Can you work these out from the model? Positions are in its coordinate system, mm. Face numbers are marked on the shaded views. A direction names the side the tool comes from. Give positions to 0.01 mm unless a question says otherwise; leave off trailing zeros. Loops run counter-clockwise (first coordinate to the right, second up) from the corner with the lowest first, then second, coordinate; pieces in that order, holes last. Notation, with made-up numbers: (-30.5, 9.25) -> (-15.5, 9.25) arc R29 cw to (-15.5, 45.25) -> close; hole circle Ø3 at (68, -5.75). An arc over 180 degrees is marked (long way). Use CSV: the item, a comma, the result in double quotes.
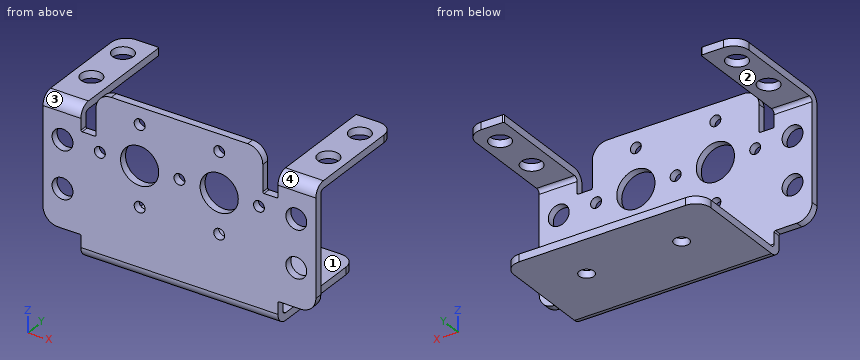
from build123d import *

# Parameters (mm, degrees)
BASE_FLANGE1_DEPTH             = 1.5494
EDGE_FLANGE1_STRIP_W           = 7.8232
EDGE_FLANGE1_STRIP_H           = 1.5494
EDGE_FLANGE1_STRIP_CUT_DEPTH   = 41.275
EDGE_FLANGE1_DEPTH             = 41.275
EDGE_FLANGE2_STRIP_W           = 7.8232
EDGE_FLANGE2_STRIP_H           = 1.5494
EDGE_FLANGE2_STRIP_CUT_DEPTH   = 7.9375
EDGE_FLANGE2_STRIP_2_W         = 7.8232
EDGE_FLANGE2_STRIP_2_H         = 1.5494
EDGE_FLANGE2_STRIP_CUT_2_DEPTH = 7.9375
EDGE_FLANGE2_DEPTH             = 7.9375
EDGE_FLANGE2_BEND_DEPTH        = 7.9375
SKETCH13_R                     = 1.143
SKETCH13_R_2                   = 4.0005
SKETCH13_R_3                   = 2.1844
EXTRUDE2_DEPTH                 = 1.5494
SKETCH14_R                     = 2.1844
EXTRUDE3_DEPTH                 = 1.5494
SKETCH15_R                     = 1.5621
EXTRUDE4_DEPTH                 = 1.5494
FILLET1_R                      = 3.175
FILLET2_R                      = 0.254


# Sheet-metal steps are written as plain solids
with BuildPart() as part:
    # Sketch1 → Base-Flange1 (new body)
    with BuildSketch(Plane(origin=(0, 0, 0), x_dir=(1, 0, 0), z_dir=(0, 1, 0))):
        Polygon((-17.4625, -11.8745), (17.4625, -11.8745), (17.4625, -2.9337), (20.6375, -2.9337), (20.6375, -6.3754), (28.575, -6.3754), (28.575, 17.8816), (20.6375, 17.8816), (20.6375, 21.3106), (-20.6375, 21.3106), (-20.6375, 17.8816), (-28.575, 17.8816), (-28.575, -6.3754), (-20.6375, -6.3754), (-20.6375, -2.9337), (-17.4625, -2.9337), align=None)
    extrude(amount=BASE_FLANGE1_DEPTH)

    # Edge-Flange1 strip (across the edge) → Edge-Flange1 strip cut (cut)
    with BuildSketch(Plane(origin=(20.6375, 1.5494, -21.3106), x_dir=(0, 0, 1), z_dir=(-1, 0, 0))):
        with Locations((-3.0988, -0.7747)):
            Rectangle(EDGE_FLANGE1_STRIP_W, EDGE_FLANGE1_STRIP_H)
    extrude(amount=EDGE_FLANGE1_STRIP_CUT_DEPTH, mode=Mode.SUBTRACT)

    # Edge-Flange1 section (across the edge) → Edge-Flange1 (add)
    with BuildSketch(Plane(origin=(20.6375, 1.5494, -21.3106), x_dir=(0, 0, 1), z_dir=(-1, 0, 0))):
        with BuildLine():
            Line((-1.5494, 0.8128), (-1.5494, 22.9108))
            Line((-1.5494, 22.9108), (0, 22.9108))
            Line((0, 22.9108), (0, 0.8128))
            ThreePointArc((0, 0.8128), (0.238063608, 0.238063608), (0.8128, 0))
            Line((0.8128, 0), (0.8128, -1.5494))
            ThreePointArc((0.8128, -1.5494), (-0.857527639, -0.857527639), (-1.5494, 0.8128))
        make_face()
    extrude(amount=EDGE_FLANGE1_DEPTH)

    # Edge-Flange2 strip (across the edge) → Edge-Flange2 strip cut (cut)
    with BuildSketch(Plane(origin=(-28.575, 1.5494, 6.3754), x_dir=(0, 0, -1), z_dir=(1, 0, 0))):
        with Locations((-3.0988, -0.7747)):
            Rectangle(EDGE_FLANGE2_STRIP_W, EDGE_FLANGE2_STRIP_H)
    extrude(amount=EDGE_FLANGE2_STRIP_CUT_DEPTH, mode=Mode.SUBTRACT)

    # Edge-Flange2 strip 2 (across the edge) → Edge-Flange2 strip cut 2 (cut)
    with BuildSketch(Plane(origin=(20.6375, 1.5494, 6.3754), x_dir=(0, 0, -1), z_dir=(1, 0, 0))):
        with Locations((-3.0988, -0.7747)):
            Rectangle(EDGE_FLANGE2_STRIP_2_W, EDGE_FLANGE2_STRIP_2_H)
    extrude(amount=EDGE_FLANGE2_STRIP_CUT_2_DEPTH, mode=Mode.SUBTRACT)

    # Edge-Flange2 section (across the edge) → Edge-Flange2 (add)
    with BuildSketch(Plane(origin=(-28.575, 1.5494, 6.3754), x_dir=(0, 0, -1), z_dir=(1, 0, 0))):
        with BuildLine():
            Line((-1.5494, 0.8128), (-1.5494, 22.9108))
            Line((-1.5494, 22.9108), (0, 22.9108))
            Line((0, 22.9108), (0, 0.8128))
            ThreePointArc((0, 0.8128), (0.238063608, 0.238063608), (0.8128, 0))
            Line((0.8128, 0), (0.8128, -1.5494))
            ThreePointArc((0.8128, -1.5494), (-0.857527639, -0.857527639), (-1.5494, 0.8128))
        make_face()
    extrude(amount=EDGE_FLANGE2_DEPTH)

    # Edge-Flange2 section 2 (across the edge) → Edge-Flange2 bend (add)
    with BuildSketch(Plane(origin=(20.6375, 1.5494, 6.3754), x_dir=(0, 0, -1), z_dir=(1, 0, 0))):
        with BuildLine():
            Line((-1.5494, 0.8128), (-1.5494, 22.9108))
            Line((-1.5494, 22.9108), (0, 22.9108))
            Line((0, 22.9108), (0, 0.8128))
            ThreePointArc((0, 0.8128), (0.238063608, 0.238063608), (0.8128, 0))
            Line((0.8128, 0), (0.8128, -1.5494))
            ThreePointArc((0.8128, -1.5494), (-0.857527639, -0.857527639), (-1.5494, 0.8128))
        make_face()
    extrude(amount=EDGE_FLANGE2_BEND_DEPTH)

    # Sketch13 → Extrude2 (cut)
    with BuildSketch(Plane(origin=(0, 1.5494, 0), x_dir=(1, 0, 0), z_dir=(0, 1, 0))):
        with Locations(Location((0, 0, 0), (0, 0, 270))):
            Circle(SKETCH13_R)
        with Locations(Location((8.3312, 8.3312, 0), (0, 0, 270))):
            Circle(SKETCH13_R)
        with Locations(Location((8.3312, -8.3312, 0), (0, 0, 270))):
            Circle(SKETCH13_R)
        with Locations(Location((16.6624, 0, 0), (0, 0, 270))):
            Circle(SKETCH13_R)
        with Locations(Location((-8.3312, 8.3312, 0), (0, 0, 270))):
            Circle(SKETCH13_R)
        with Locations(Location((-8.3312, -8.3312, 0), (0, 0, 270))):
            Circle(SKETCH13_R)
        with Locations(Location((-16.6624, 0, 0), (0, 0, 270))):
            Circle(SKETCH13_R)
        with Locations(Location((-8.3312, 0, 0), (0, 0, 270))):
            Circle(SKETCH13_R_2)
        with Locations(Location((8.3312, 0, 0), (0, 0, 270))):
            Circle(SKETCH13_R_2)
        with Locations(Location((-24.4856, 9.8552, 0), (0, 0, 270))):
            Circle(SKETCH13_R_3)
        with Locations(Location((-24.4856, 0, 0), (0, 0, 270))):
            Circle(SKETCH13_R_3)
        with Locations(Location((24.4856, 9.8552, 0), (0, 0, 270))):
            Circle(SKETCH13_R_3)
        with Locations(Location((24.4856, 0, 0), (0, 0, 270))):
            Circle(SKETCH13_R_3)
    extrude(amount=-EXTRUDE2_DEPTH, mode=Mode.SUBTRACT)

    # Sketch14 → Extrude3 (cut)
    with BuildSketch(Plane.XY.offset(7.9248)):
        with Locations((-24.8158, 19.3802)):
            Circle(SKETCH14_R)
        with Locations((-24.8158, 9.525)):
            Circle(SKETCH14_R)
        with Locations((24.8158, 19.3802)):
            Circle(SKETCH14_R)
        with Locations((24.8158, 9.525)):
            Circle(SKETCH14_R)
    extrude(amount=-EXTRUDE3_DEPTH, mode=Mode.SUBTRACT)

    # Sketch15 → Extrude4 (cut)
    with BuildSketch(Plane(origin=(0, 0, -22.86), x_dir=(-1, 0, 0), z_dir=(0, 0, -1))):
        with Locations(Location((-9.9441, 14.5161, 0), (0, 0, 90))):
            Circle(SKETCH15_R)
        with Locations(Location((9.9441, 14.5161, 0), (0, 0, 90))):
            Circle(SKETCH15_R)
    extrude(amount=-EXTRUDE4_DEPTH, mode=Mode.SUBTRACT)

    # Fillet1
    fillet1_edges = [part.edges().sort_by_distance(p)[0] for p in [
        (-28.575, 24.4602, 7.1501),
        (28.575, 24.4602, 7.1501),
        (-28.575, 0.7747, -17.8816),
        (28.575, 0.7747, -17.8816),
        (17.4625, 0.7747, 11.8745),
        (-17.4625, 0.7747, 11.8745),
        (20.6375, 24.4602, -22.0853),
        (-20.6375, 24.4602, -22.0853),
    ]]
    fillet(fillet1_edges, radius=FILLET1_R)

    # Fillet2
    fillet2_edges = [part.edges().sort_by_distance(p)[0] for p in [
        (-20.6375, 24.4602, 7.1501),
        (20.6375, 24.4602, 7.1501),
        (-17.4625, 0.7747, 2.9337),
        (-20.6375, 0.7747, 2.9337),
        (-20.6375, 0.7747, -17.8816),
        (20.6375, 0.7747, -17.8816),
        (20.6375, 0.7747, 2.9337),
        (17.4625, 0.7747, 2.9337),
    ]]
    fillet(fillet2_edges, radius=FILLET2_R)


solid = part.part
(1) If we section it at C-C, the plane y = 5: Write out the boundary of the cut face in (x, z) (1 decimal).
Answer sheet:
outline,"(-28.6, 6.4) -> (-20.6, 6.4) -> (-20.6, 7.9) -> (-28.6, 7.9) -> close; (-20.6, -22.9) -> (20.6, -22.9) -> (20.6, -21.3) -> (-20.6, -21.3) -> close; (20.6, 6.4) -> (28.6, 6.4) -> (28.6, 7.9) -> (20.6, 7.9) -> close"
(2) If we section it at A-A, the plane x = 0: Write out the boundary of the cut face in (y, z).
Answer sheet:
outline,"(0, -20.5) arc R2.36 ccw to (2.36, -22.86) -> (24.46, -22.86) -> (24.46, -21.31) -> (2.36, -21.31) arc R0.81 cw to (1.55, -20.5) -> (1.55, -1.14) -> (0, -1.14) -> close; (0, 1.14) -> (1.55, 1.14) -> (1.55, 11.87) -> (0, 11.87) -> close"
(3) If we section it at B-B, the plane z = 0: Give the number of separate pieces and of enclosed holes in the cut face, then the cut area to 3 significant figures.
Answer sheet:
separate pieces,"8"
enclosed holes,"0"
area,"39.6 mm2"
(4) Will these pins go through, and if not, where does the flat tip stop? pin 1 Ø5 at (x, y) = (-2, 13) entering from +Z; pin 2 Ø5.5 at (x, y) = (24.82, 19.38) entering from -Z; pin 3 Ø2.5 at (x, z) = (-16.66, 0) entering from +Y.
Answer sheet:
pin 1,"stops at z = -21.31"
pin 2,"stops at z = 6.38"
pin 3,"stops at y = 1.55"
(5) Which directions (+Z, -Z, +X, -X, +Y, -Y) give clear straight access to the entire face, cutting with the end or side of a thin tool? Please do the marked faces 1, 2, 3 and 4.
Answer sheet:
face 1,"+Z, +X, -X, +Y"
face 2,"-Z, +X, -X, +Y"
face 3,"+Z, -X, -Y"
face 4,"+Z, +X, -Y"
(6) If we section it at D-D, the plane z = -5.5: Write out the boundary of the cut face in (x, y) (3 decimals).
Answer sheet:
outline,"(-28.575, 0) -> (28.575, 0) -> (28.575, 1.549) -> (-28.575, 1.549) -> close"
(7) If I drill on L1, parallel to X at y = 15, z = 7.5 (1 decimal); L2, parallel to Y at x = 2, z = -1.5; L3, parallel to Z at x = -2.5, y = 17.25, over which ranges is the centre line in solid material (lowest first)? Write a range as from..to.
Answer sheet:
L1,"x = -28.6..-20.6, 20.6..28.6"
L2,"y = 0..1.55"
L3,"z = -22.86..-21.31"
